Geometry check sheet. Reference: the model listing, model coordinates, mm. A direction names the side the tool comes from. Give positions to 0.01 mm unless a question says otherwise; leave off trailing zeros. Order: outer loops, then holes, each group sorted by start corner. A loop starts at its lowest first (then second) coordinate and runs counter-clockwise, first axis right, second up. Notation, with made-up numbers: M 4.5,51 L 59.5,51 A30 ccw 59.5,86 Z; hole C -8,56.25 d8. An arc over 180 degrees is marked long. One line per question, with ' | ' between items. Start each with the question number.
from build123d import *

# Parameters (mm, degrees)
TUBO_TIJA_PROFILE_R         = 13.6
CABEZA_PROFILE_R            = 10
VACIADO_TUBO_TIJA_PROFILE_R = 11.6


with BuildPart() as part:
    # Tubo_tija: sweep along a curve in space
    with BuildLine() as tubo_tija_path:
        Line((-115.633009218, 378.218530983, 0), (-197.165716473, 644.9, 0))
    # Tubo_tija profile (on start of the path) → Tubo_tija (sweep)
    with BuildSketch(Plane(origin=(-115.633009218, 378.218530983, 0), x_dir=(0.9563047559630354, 0.2923717047227369, 0), z_dir=(-0.2923717047227369, 0.9563047559630354, 0))):
        Circle(TUBO_TIJA_PROFILE_R)
    sweep(path=tubo_tija_path.line)

    # Cabeza: sweep along a curve in space
    with BuildLine() as cabeza_path:
        Line((-197.165716473, 644.9, -25), (-197.165716473, 644.9, 25))
    # Cabeza profile (on start of the path) → Cabeza (sweep)
    with BuildSketch(Plane(origin=(-197.165716473, 644.9, -25), x_dir=(1, 0, 0), z_dir=(0, 0, 1))):
        Circle(CABEZA_PROFILE_R)
    sweep(path=cabeza_path.line)

    # Vaciado_Tubo_tija: sweep along a curve in space
    with BuildLine() as vaciado_tubo_tija_path:
        Line((-115.633009218, 378.218530983, 0), (-197.165716473, 644.9, 0))
    # Vaciado_Tubo_tija profile (on start of the path) → Vaciado_Tubo_tija (sweep, cut)
    with BuildSketch(Plane(origin=(-115.633009218, 378.218530983, 0), x_dir=(0.9563047559630354, 0.2923717047227369, 0), z_dir=(-0.2923717047227369, 0.9563047559630354, 0))):
        Circle(VACIADO_TUBO_TIJA_PROFILE_R)
    sweep(path=vaciado_tubo_tija_path.line, mode=Mode.SUBTRACT)


solid = part.part
Item 1: Cross-section at A-A, the plane z = 3. Record the cut outline in (x, y).
Item 2: Set-up check for faces 5 (the cylindrical face through (-198.468, 654.815, 0.35)), 6 (the flat face through (-197, 645, 25)): record each of +Z, -Z, +X, -X, +Y, -Y from which the full face is reachable in a straight line by a thin tool's end or side.
Item 3: Material ranges on line 1 along Z through (x, y) = (-190, 624.5); line 2 along X through (y, z) = (418, -1); line 3 along Z through (x, y) = (-173.5, 574), recorded low to high.
Item 4: Cross-section at B-B, the plane z = 19.5. Record the cut outline in (x, y), plus the area to 3 significant figures.
Item 5: Depth check by flat-ended pin: pin 1 (12 mm diameter, centred on y = 485.5, z = 4.5, fed in from -X); pin 2 (3 mm diameter, centred on x = -166.5, y = 590, fed in from +Z). Enter the tip coordinate at first touch or a pass-through.
Item 6: Mould release check, pull along X, two halves, no side actions. Record for faces 1 (the flat face through (-197.3, 644.86, -0.16)), 2 (the cylindrical face through (-169.96, 509.45, -0.6)), 3 (the flat face through (-197, 645, -25)), 4 (the flat face through (-105.096, 381.44, -4.093)): released by +X, released by -X, zero draft, split by the parting line, or undercut.
Outcome:
1) outline: M -209.85,641.02 L -128.32,374.34 L -126.35,374.94 L -207.88,641.62 Z; M -206.73,641.98 L -187.6,647.82 A10 ccw Z; M -186.45,648.18 L -104.92,381.49 L -102.95,382.1 L -184.48,648.78 Z
2) face 5: none | face 6: +Z, +X, -X, +Y, -Y
3) line 1: z = -13.57 to -11.57, 11.57 to 13.57 | line 2: x = -141.98 to -139.88, -115.71 to -113.61 | line 3: z = -13.47 to -11.44, 11.44 to 13.47
4) outline: C -197.17,644.9 d20 | area: 314 mm²
5) pin 1: stops at x = -164.17 | pin 2: stops at z = 6.81
6) face 1: undercut | face 2: split by the parting line | face 3: zero draft | face 4: released by +X
